The model under review builds one solid part; all positions refer to its coordinate system, in mm. A direction names the side the tool comes from. Give positions to 0.01 mm unless a question says otherwise; leave off trailing zeros. Order: outer loops, then holes, each group sorted by start corner. A loop starts at its lowest first (then second) coordinate and runs counter-clockwise, first axis right, second up. Notation, with made-up numbers: (69.5, 77.5) - (77.5, 77.5) arc R17 ccw to (77.5, 106.5) - close; hole circle Ø9 at (46.25, 3.25). An arc over 180 degrees is marked (long way). Use a Markdown table: item, result. Add a question column.
```python
from build123d import *

# Parameters (mm, degrees)
PAD_DEPTH    = 10
PAD001_DEPTH = 10
PAD002_DEPTH = 37
PAD003_DEPTH = 2
FILLET_R     = 0.5


with BuildPart() as part:
    # Sketch → Pad (new body)
    with BuildSketch(Plane.XY):
        with BuildLine():
            ThreePointArc((7.487957, -6.322222), (0, 9.8), (-7.487957, -6.322222))
            ThreePointArc((-7.539231, -7.539231), (-7.276425, -6.940719), (-7.487957, -6.322222))
            Line((-7.823043, -7.823043), (-7.539231, -7.539231))
            ThreePointArc((-9.145339, -7.769348), (-8.495956, -8.085906), (-7.823043, -7.823043))
            ThreePointArc((9.145339, -7.769348), (0, 12), (-9.145339, -7.769348))
            ThreePointArc((7.823043, -7.823043), (8.495956, -8.085906), (9.145339, -7.769348))
            Line((7.539231, -7.539231), (7.823043, -7.823043))
            ThreePointArc((7.487957, -6.322222), (7.276425, -6.940719), (7.539231, -7.539231))
        make_face()
    extrude(amount=PAD_DEPTH)

    # Sketch001 → Pad001 (join)
    with BuildSketch(Plane.XY):
        with BuildLine():
            Line((-6.63325, 15), (6.63325, 15))
            Line((6.63325, 15), (6.63325, 10))
            ThreePointArc((6.63325, 10), (0, 12), (-6.63325, 10))
            Line((-6.63325, 10), (-6.63325, 15))
        make_face()
    extrude(amount=PAD001_DEPTH)

    # Sketch002 → Pad002 (join)
    with BuildSketch(Plane.XY):
        with BuildLine():
            ThreePointArc((-13.957974, 47.773263), (0, 16.130227), (13.957974, 47.773263))
            ThreePointArc((13.986243, 49.01647), (13.722872, 48.400534), (13.957974, 47.773263))
            Line((13.986243, 49.01647), (14.269373, 49.2996))
            ThreePointArc((15.569887, 49.270614), (14.925823, 49.56298), (14.269373, 49.2996))
            ThreePointArc((-15.569887, 49.270614), (0, 13.930227), (15.569887, 49.270614))
            ThreePointArc((-14.269373, 49.2996), (-14.925823, 49.56298), (-15.569887, 49.270614))
            Line((-14.269373, 49.2996), (-13.986243, 49.01647))
            ThreePointArc((-13.957974, 47.773263), (-13.722872, 48.400534), (-13.986243, 49.01647))
        make_face()
    extrude(amount=PAD002_DEPTH)

    # Sketch003 → Pad003 (join)
    with BuildSketch(Plane.XY):
        with BuildLine():
            Line((6.63325, 15), (6.63325, 35))
            ThreePointArc((6.63325, 35), (5.461677, 37.828427), (2.63325, 39))
            Line((2.63325, 39), (-2.63325, 39))
            ThreePointArc((-2.63325, 39), (-5.461677, 37.828427), (-6.63325, 35))
            Line((-6.63325, 35), (-6.63325, 15))
            Line((-6.63325, 15), (6.63325, 15))
        make_face()
    extrude(amount=PAD003_DEPTH)

    # Fillet
    fillet_edges = [part.edges().sort_by_distance(p)[0] for p in [
        (0, 9.8, 10),
        (11.881852, 1.679762, 10),
        (-11.881852, 1.679762, 10),
        (0, 13.930227, 37),
        (0, 16.130227, 37),
    ]]
    fillet(fillet_edges, radius=FILLET_R)


solid = part.part
```
Q1. Clearance check with flat-ended pins moving along their axes: P1, Ø3, axis at y = 12.5, z = 3.5, coming from the +X side; P2, Ø15.5, axis at x = 0, y = 0, coming from the -Z side; P3, Ø2, axis at y = 22, z = 28.5, coming from the +X side; P4, Ø25, axis at x = 2.5, y = -0.5, coming from the +Z side. State where each tip first meets the part, or that it passes through.
Q2. We need section B-B (z = 18). Write out the cut boundary in (x, y), plus the area to 3 significant figures.
Q3. Machinability: for faces 4 (the flat face through (-6, 16, 37)), 5 (the flat face through (-6.633, 26, 1)), 6 (the cylindrical face through (-13.723, 48.391, 17.994)), 7 (the flat face through (0, 28, 2)), 8 (the cylindrical face through (8.486, -8.086, 4.684)), which of the approach directions +Z, -Z, +X, -X, +Y, -Y give a long, thin tool a straight path to every point of the face, cutting with its end or side? Answer none if there is none.
Q4. Draft analysis for pull direction X (two halves, no side actions). For faces 1 (the cylindrical face through (11.9, 1.54, 4.68)), 2 (the flat face through (-6.633, 12, 5)), 3 (the cylindrical face through (7.276, -6.931, 4.684)), state which applies: pulls with the +X half, pulls with the -X half, needs draft (parallel to the pull), parting line crosses it, or undercut.
Q5. Wall thickness on probe 1 along X at (y, z) = (34.5, 19.5); probe 2 along Y at (x, z) = (0, 2.5); probe 3 along X at (y, z) = (6.5, 7.5): over which ranges is each line inside the solid? List them lowest first.
Q6. We need section C-C (y = 32). Count the separate pieces of the cut face and the enclosed holes in it, plus the area to 3 significant figures.
Q7. We need section A-A (x = 0). Write out the cut boundary in (y, z).
Here are the results:
| question | item | result |
|---|---|---|
| 1 | P1 | x = 6.63 |
| 1 | P2 | through |
| 1 | P3 | x = 17.33 |
| 1 | P4 | z = 10 |
| 2 | outline | (-15.57, 49.27) arc R21.1 ccw (long way) to (15.57, 49.27) arc R0.9 ccw to (14.27, 49.3) - (13.99, 49.02) arc R0.9 ccw to (13.96, 47.77) arc R18.9 cw (long way) to (-13.96, 47.77) arc R0.9 ccw to (-13.99, 49.02) - (-14.27, 49.3) arc R0.9 ccw to start |
| 2 | area | 207 mm2 |
| 3 | face 4 | +Z, +X, -X, +Y, -Y |
| 3 | face 5 | +Z, -Z, +Y |
| 3 | face 6 | +Z, -Z |
| 3 | face 7 | +Z, +Y |
| 3 | face 8 | +Z, -Z, -Y |
| 4 | face 1 | pulls with the +X half |
| 4 | face 2 | pulls with the -X half |
| 4 | face 3 | undercut |
| 5 | probe 1 | -21.09 to -18.89, 18.89 to 21.09 |
| 5 | probe 2 | 9.8 to 16.13 |
| 5 | probe 3 | -10.09 to -7.33, 7.33 to 10.09 |
| 6 | separate pieces | 3 |
| 6 | enclosed holes | 0 |
| 6 | area | 191 mm2 |
| 7 | outline | (9.8, 0) - (39, 0) - (39, 2) - (16.13, 2) - (16.13, 36.5) arc R0.5 ccw to (15.63, 37) - (14.43, 37) arc R0.5 ccw to (13.93, 36.5) - (13.93, 10) - (10.3, 10) arc R0.5 ccw to (9.8, 9.5) - close |
